```python
from build123d import *

# Parameters (mm, degrees)
F0_W      = 25
F0_H      = 25
F1_DEPTH  = 30
F3_DEPTH  = 25.001
F4_R      = 2.1
F5_DEPTH  = 25.001
F6_R      = 5
F7_DEPTH  = 22
F9_DEPTH  = 7
F10_R     = 2.6
F11_DEPTH = 15


with BuildPart() as f1:
    # F0 (on Right) → F1 (new body, symmetric)
    with BuildSketch(Plane.YZ):
        Rectangle(F0_W, F0_H)
    extrude(amount=F1_DEPTH, both=True)

    # F2 (on face) → F3 (cut, through all)
    with BuildSketch(Plane.XY.offset(12.5)):
        with BuildLine():
            Line((12, -12.5), (22, -12.5))
            ThreePointArc((22, -12.5), (17, -7.5), (12, -12.5))
        make_face()
    extrude(amount=-F3_DEPTH, mode=Mode.SUBTRACT)

    # F4 (on face) → F5 (cut, through all)
    with BuildSketch(Plane.XY.offset(12.5)):
        with Locations((17, -4.5)):
            Circle(F4_R)
    extrude(amount=-F5_DEPTH, mode=Mode.SUBTRACT)

    # F6 (on face) → F7 (cut)
    with BuildSketch(Plane(origin=(0, 0, -12.5), x_dir=(1, 0, 0), z_dir=(0, 0, -1))):
        with Locations((5, 5.5)):
            Circle(F6_R)
    extrude(amount=-F7_DEPTH, mode=Mode.SUBTRACT)

    # F8 (on face) → F9 (cut)
    with BuildSketch(Plane.XZ.offset(12.5)):
        with BuildLine():
            Line((1.5, -12.5), (8.5, -12.5))
            Line((8.5, -12.5), (8.5, 2.5))
            ThreePointArc((8.5, 2.5), (5, 6), (1.5, 2.5))
            Line((1.5, 2.5), (1.5, -12.5))
        make_face()
    extrude(amount=-F9_DEPTH, mode=Mode.SUBTRACT)

    # F10 (on face) → F11 (cut)
    with BuildSketch(Plane(origin=(0, 0, -12.5), x_dir=(1, 0, 0), z_dir=(0, 0, -1))):
        with Locations((17, 4.5)):
            Circle(F10_R)
    extrude(amount=-F11_DEPTH, mode=Mode.SUBTRACT)


with BuildPart() as f12_1:
    # F12: copy of F1
    add(f1.part)


solid = f1.part
```
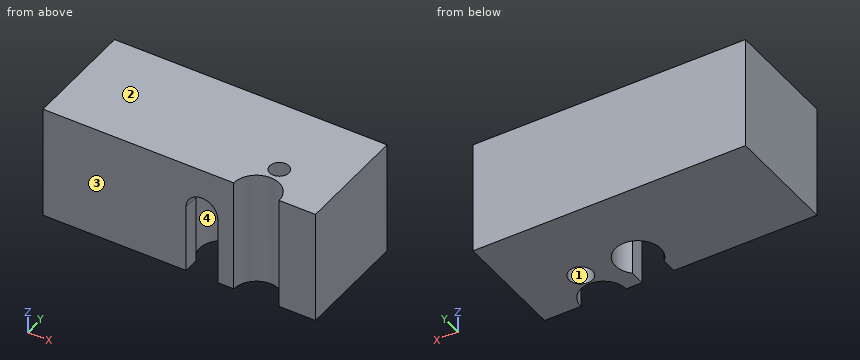
Model file for the job. Use its own axes, mm. Face numbers are marked on the shaded views. Give positions to 0.01 mm unless a question says otherwise; leave off trailing zeros. Write each loop counter-clockwise with the first axis right and the second up, starting at its lowest first coordinate (ties: lowest second). Pieces come first, ordered by that corner, then holes. Notation, with made-up numbers: (-24, 40) -> (21, 40) arc R16 cw to (21, 54) -> close; hole circle Ø8 at (57.25, 49.25). An arc over 180 degrees is marked (long way). Use CSV: the item, a comma, the result in double quotes. Start each with the question number.
1) Drill centre lines: L1, parallel to Y at x = 17, z = -5; L2, parallel to X at y = -5.5, z = 1.75; L3, parallel to X at y = -4.5, z = -6. Where is each one in solid material? Low to high.
2) Cut at B-B on y = -3.5. List the corners of the cut face in (x, z), plus the area to 3 significant figures.
3) Two-plate mould, pull along Y, no slides. Class the marked faces 1, 2, 3 and 4: released by +Y, released by -Y, zero draft, split by the parting line, or undercut.
4) Pin check, flat tips, straight feed: P1, Ø8.5, axis at x = 17, y = -4.5, coming from the -Z side; P2, Ø4, axis at x = 17, y = -4.5, coming from the -Z side; P3, Ø2.5, axis at x = 17.5, y = -3.5, coming from the -Z side; P4, Ø5, axis at x = 4.5, z = -2, coming from the -Y side. Stop position of each tip, or through.
5) Cut at C-C on x = 5. List the corners of the cut face in (y, z), plus the area to 3 significant figures.
6) Cut at A-A on x = 17. List the corners of the cut face in (y, z).
Final values:
1,L1,"y = -7.5 to -7.1, -1.9 to 12.5"
1,L2,"x = -30 to 0, 10 to 14.6, 19.4 to 30"
1,L3,"x = -30 to 0.1, 9.9 to 14.4, 19.6 to 30"
2,outline,"(-30, -12.5) -> (0.42, -12.5) -> (0.42, 9.5) -> (9.58, 9.5) -> (9.58, -12.5) -> (14.6, -12.5) -> (14.6, 2.5) -> (15.15, 2.5) -> (15.15, 12.5) -> (-30, 12.5) -> close; (18.85, 2.5) -> (19.4, 2.5) -> (19.4, -12.5) -> (30, -12.5) -> (30, 12.5) -> (18.85, 12.5) -> close"
2,area,"1,190 mm2"
3,face 1,"undercut"
3,face 2,"zero draft"
3,face 3,"released by -Y"
3,face 4,"undercut"
4,P1,"stops at z = -12.5"
4,P2,"passes through"
4,P3,"stops at z = 2.5"
4,P4,"stops at y = -1.5"
5,outline,"(-12.5, 6) -> (-10.5, 6) -> (-10.5, 9.5) -> (-0.5, 9.5) -> (-0.5, -12.5) -> (12.5, -12.5) -> (12.5, 12.5) -> (-12.5, 12.5) -> close"
5,area,"368 mm2"
6,outline,"(-7.5, -12.5) -> (-7.1, -12.5) -> (-7.1, 2.5) -> (-6.6, 2.5) -> (-6.6, 12.5) -> (-7.5, 12.5) -> close; (-2.4, 2.5) -> (-1.9, 2.5) -> (-1.9, -12.5) -> (12.5, -12.5) -> (12.5, 12.5) -> (-2.4, 12.5) -> close"
